Model file for the job. Use its own axes, mm. A direction names the side the tool comes from. Give positions to 0.01 mm unless a question says otherwise; leave off trailing zeros. Write each loop counter-clockwise with the first axis right and the second up, starting at its lowest first coordinate (ties: lowest second). Pieces come first, ordered by that corner, then holes.
```python
from build123d import *

# Parameters (mm, degrees)
SALIENTE_EXTRUIR1_DEPTH    = 25
CORTAR_EXTRUIR1_START      = -94
CROQUIS2_R                 = 9.5
CORTAR_EXTRUIR1_DEPTH      = 148
CROQUIS3_R                 = 15
CROQUIS3_R_2               = 16
CORTAR_EXTRUIR2_DEPTH      = 94
CORTAR_EXTRUIR3_DEPTH      = 94
CHAFL_N2_SIZE              = 5
SALIENTE_EXTRUIR2_DEPTH    = 17
CHAFL_N2_OF_SIMETR_A1_SIZE = 5
CROQUIS6_W                 = 120.154705919
CROQUIS6_H                 = 59.700185721
CORTAR_EXTRUIR4_DEPTH      = 90


with BuildPart() as part:
    # Croquis1 → Saliente-Extruir1 (new body)
    with BuildSketch(Plane(origin=(0, 0, 0), x_dir=(0, 0, -1), z_dir=(1, 0, 0))):
        Polygon((-100, 0), (-82, 40), (0, 40), (0, 0), align=None)
    saliente_extruir1 = extrude(amount=SALIENTE_EXTRUIR1_DEPTH)

    # Croquis2 → Cortar-Extruir1 (cut)
    with BuildSketch(Plane(origin=(0, 40, 0), x_dir=(1, 0, 0), z_dir=(0, 1, 0)).offset(CORTAR_EXTRUIR1_START)):
        with Locations((13, -100)):
            Circle(CROQUIS2_R)
        with Locations(Location((13, -20, 0), (0, 0, 90))):
            Circle(CROQUIS2_R)
    cortar_extruir1 = extrude(amount=CORTAR_EXTRUIR1_DEPTH, mode=Mode.SUBTRACT)

    # Croquis3 → Cortar-Extruir2 (cut, symmetric)
    with BuildSketch(Plane(origin=(25, 0, 0), x_dir=(0, 0, -1), z_dir=(1, 0, 0))):
        with Locations((-35, 40)):
            Circle(CROQUIS3_R)
        with Locations((-63, 0)):
            Circle(CROQUIS3_R_2)
    cortar_extruir2 = extrude(amount=CORTAR_EXTRUIR2_DEPTH, both=True, mode=Mode.SUBTRACT)

    # Croquis4 → Cortar-Extruir3 (cut, symmetric)
    with BuildSketch(Plane(origin=(0, 40, 0), x_dir=(1, 0, 0), z_dir=(0, 1, 0))):
        Polygon((12.62, 0), (25, -13.066583333), (25, 0), align=None)
    cortar_extruir3 = extrude(amount=CORTAR_EXTRUIR3_DEPTH, both=True, mode=Mode.SUBTRACT)

    # Chafl_n2
    chafl_n2_edges = [part.edges().sort_by_distance(p)[0] for p in [
        (0, 20, 0),
    ]]
    chamfer(chafl_n2_edges, length=CHAFL_N2_SIZE)

    # Croquis5 → Saliente-Extruir2 (add)
    with BuildSketch(Plane(origin=(25, 0, 0), x_dir=(0, 0, -1), z_dir=(1, 0, 0))):
        with BuildLine():
            Line((-87.5, 0), (-83, 0))
            ThreePointArc((-83, 0), (-63, 20), (-43, 0))
            Line((-43, 0), (-38.5, 0))
            ThreePointArc((-38.5, 0), (-63, 24.5), (-87.5, 0))
        make_face()
    saliente_extruir2 = extrude(amount=SALIENTE_EXTRUIR2_DEPTH)


with BuildPart() as simetr_a1_1:
    # Simetr_a1: Saliente-Extruir1 across plane
    add(saliente_extruir1.mirror(Plane(origin=(0, 0, 0), x_dir=(0, 0, 1), z_dir=(1, 0, 0))))

    # Simetr_a1 2: Cortar-Extruir1, Cortar-Extruir2, Cortar-Extruir3 across plane
    add(cortar_extruir1.mirror(Plane(origin=(0, 0, 0), x_dir=(0, 0, 1), z_dir=(1, 0, 0))), mode=Mode.SUBTRACT)
    add(cortar_extruir2.mirror(Plane(origin=(0, 0, 0), x_dir=(0, 0, 1), z_dir=(1, 0, 0))), mode=Mode.SUBTRACT)
    add(cortar_extruir3.mirror(Plane(origin=(0, 0, 0), x_dir=(0, 0, 1), z_dir=(1, 0, 0))), mode=Mode.SUBTRACT)

    # Chafl_n2 of Simetr_a1
    chafl_n2_of_simetr_a1_edges = [simetr_a1_1.edges().sort_by_distance(p)[0] for p in [
        (0, 20, 0),
    ]]
    chamfer(chafl_n2_of_simetr_a1_edges, length=CHAFL_N2_OF_SIMETR_A1_SIZE)


with BuildPart() as simetr_a1_3_1:
    # Simetr_a1 3: Saliente-Extruir2 across plane
    add(saliente_extruir2.mirror(Plane(origin=(0, 0, 0), x_dir=(0, 0, 1), z_dir=(1, 0, 0))))


with BuildPart() as part_1:
    add(part.part)

    # Simetr_a1 united with what the copies to: union Simetr_a1_1, Simetr_a1 3_1
    add(simetr_a1_1.part)
    add(simetr_a1_3_1.part)

    # Croquis6 → Cortar-Extruir4 (cut)
    with BuildSketch(Plane(origin=(0, 0, 0), x_dir=(0, 0, -1), z_dir=(1, 0, 0))):
        with Locations((-45.74339831, 19.581609369)):
            Rectangle(CROQUIS6_W, CROQUIS6_H)
    extrude(amount=CORTAR_EXTRUIR4_DEPTH, mode=Mode.SUBTRACT)


solid = part_1.part
```
1. Pull direction Z, two halves, no side cores. Call faces 1 (the cylindrical face through (-33, 20, 63)), 2 (the flat face through (-3, 20, 2)), 3 (the flat face through (0, 20, 53)): +Z half, -Z half, draft (parallel to the pull), parting line (faces both ways), or undercut.
Calculated:
face 1: undercut
face 2: -Z half
face 3: draft
2. Slice it at A-A, the plane y = 5.5. Write the cut outline in (x, z) (3 decimals).
Calculated:
outline: (-42, 39.125) - (-25, 39.125) - (-25, 13.067) - (-12.62, 0) - (-5, 0) - (0, 5) - (0, 47.975) - (-25, 47.975) - (-25, 43.771) - (-42, 43.771) - close; (-42, 82.229) - (-25, 82.229) - (-25, 78.025) - (0, 78.025) - (0, 97.525) - (-3.828, 97.525) arc R9.5 cw to (-22.172, 97.525) - (-25, 97.525) - (-25, 86.875) - (-42, 86.875) - close; hole circle Ø19 at (-13, 20)
3. Slice it at D-D, the plane y = 34. Write the cut outline in (x, z).
Calculated:
outline: (-25, 13.07) - (-12.62, 0) - (-5, 0) - (0, 5) - (0, 21.25) - (-3.58, 21.25) arc R9.5 cw (long way) to (-22.42, 21.25) - (-25, 21.25) - close; (-25, 48.75) - (0, 48.75) - (0, 84.7) - (-25, 84.7) - close
4. Slice it at C-C, the plane z = 94.5. Write the cut outline in (x, y).
Calculated:
outline: (-25, 0) - (-20.75, 0) - (-20.75, 12.22) - (-25, 12.22) - close; (-5.25, 0) - (0, 0) - (0, 12.22) - (-5.25, 12.22) - close
5. Slice it at B-B, the plane x = -15. Write the cut outline in (y, z), and give its area (3 significant figures).
Calculated:
outline: (0, 2.51) - (40, 2.51) - (40, 10.71) - (0, 10.71) - close; (0, 29.29) - (26.13, 29.29) arc R15 cw to (40, 50) - (40, 82) - (20.64, 90.71) - (0, 90.71) - (0, 79) arc R16 cw to (0, 47) - close
area: 2,040 mm2
6. Pin check, flat tips, straight feed: P1, Ø2, axis at x = -23.5, y = 10.5, coming from the -Z side; P2, Ø3, axis at x = -17.5, y = 16, coming from the -Z side; P3, Ø10, axis at x = -23.5, y = 25.5, coming from the -Z side. Stop position of each tip, or through.
Calculated:
P1: stops at z = 10.43
P2: stops at z = 3.57
P3: stops at z = 6.21
7. Which spindle directions (+Z, -Z, +X, -X, +Y, -Y) get a long thin tool onto all of the face, cutting with end or side? Do faces 4 (the flat face through (-10, 40, 8)), 5 (the cylindrical face through (-33.381, 24.494, 62.461)), 6 (the flat face through (-25, 16, 66)). Say none if no direction does.
Calculated:
face 4: +Z, -Z, +X, -X, +Y
face 5: -X, +Y
face 6: -X, -Y
8. Probe probe 1 along X at (y, z) = (10, 20); probe 2 along Z at (x, y) = (-24, 7); probe 3 along Z at (x, y) = (-32, 3). List the from-to ranges inside material, lowest first.
Calculated:
probe 1: x = -25 to -22.5, -3.5 to 0
probe 2: z = 12.01 to 48.61, 77.39 to 96.85
probe 3: z = 38.68 to 43.23, 82.77 to 87.32
